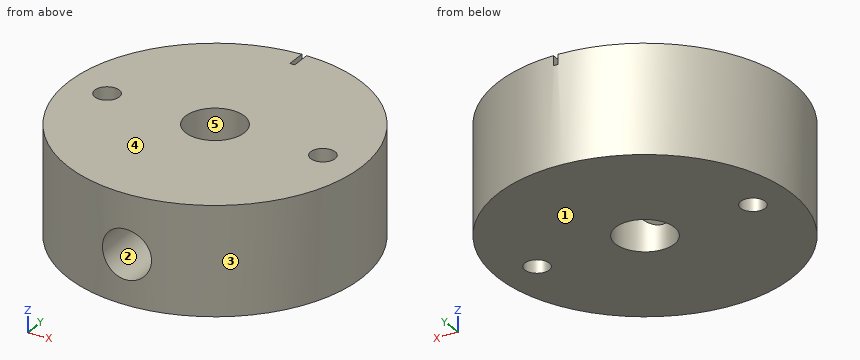
from build123d import *

# Parameters (mm, degrees)
CROQUIS1_R              = 15
CROQUIS1_R_2            = 3
SALIENTE_EXTRUIR1_DEPTH = 11
CORTAR_EXTRUIR1_START   = -1
CORTAR_EXTRUIR1_DEPTH   = 1
CROQUIS3_R              = 1.25
CORTAR_EXTRUIR2_DEPTH   = 24.895606291
CROQUIS4_R              = 2.5
CORTAR_EXTRUIR3_DEPTH   = 16


# Read off the part's stored shape, not the designer's step: Cortar-Extruir1
with BuildPart() as part:
    # Croquis1 → Saliente-Extruir1 (new body)
    with BuildSketch(Plane.XY):
        Circle(CROQUIS1_R)
        Circle(CROQUIS1_R_2, mode=Mode.SUBTRACT)
    extrude(amount=SALIENTE_EXTRUIR1_DEPTH)

    # Cortar-Extruir1 outline → Cortar-Extruir1 (cut)
    with BuildSketch(Plane.XY.offset(11).offset(CORTAR_EXTRUIR1_START)):
        with BuildLine():
            Line((-0.25, 14.997916522), (-0.25, 12.997916522))
            Line((-0.25, 12.997916522), (0.25, 12.997916522))
            Line((0.25, 12.997916522), (0.25, 14.997916522))
            ThreePointArc((0.25, 14.997916522), (0, 15), (-0.25, 14.997916522))
        make_face()
    extrude(amount=CORTAR_EXTRUIR1_DEPTH, mode=Mode.SUBTRACT)

    # Croquis3 → Cortar-Extruir2 (cut, through all)
    with BuildSketch(Plane.XY.offset(11)):
        with Locations((11, 0)):
            Circle(CROQUIS3_R)
        with Locations((-11, 0)):
            Circle(CROQUIS3_R)
    extrude(amount=-CORTAR_EXTRUIR2_DEPTH, mode=Mode.SUBTRACT)

    # Croquis4 → Cortar-Extruir3 (cut)
    with BuildSketch(Plane(origin=(0, 0, 0), x_dir=(1, 0, 0), z_dir=(0, 1, 0))):
        with Locations(Location((0, -5, 0), (0, 0, 270))):
            Circle(CROQUIS4_R)
    extrude(amount=-CORTAR_EXTRUIR3_DEPTH, mode=Mode.SUBTRACT)


solid = part.part
Build history of the part. All positions in model axes, mm. Face numbers are marked on the shaded views. A direction names the side the tool comes from. Coordinates: 2 decimals unless noted, no trailing zeros. Write each loop counter-clockwise with the first axis right and the second up, starting at its lowest first coordinate (ties: lowest second). Pieces come first, ordered by that corner, then holes.
(1) Cut at D-D on z = 5. List the corners of the cut face in (x, y).
(2) Mould opens along Y. For the marked faces 3, 4 and 5 say: pulls with the +Y half, pulls with the -Y half, needs draft (parallel to the pull), parting line crosses it, or undercut.
(3) Pin check, flat tips, straight feed: pin 1 Ø2 at (x, y) = (-9.5, 5) entering from -Z; pin 2 Ø0.8 at (y, z) = (14, 10.5) entering from -X; pin 3 Ø1.1 at (y, z) = (14, 10.5) entering from +X; pin 4 Ø5 at (y, z) = (4.5, 5) entering from +X. Stop position of each tip, or through.
(4) 3-axis set-ups, long thin cutter, end or side, ignore diameter. For the marked faces 1 and 2: which of +Z, -Z, +X, -X, +Y, -Y reach the whole face in a straight line?
(5) Cut at B-B on x = 1.5. List the corners of the cut face in (y, z).
(6) Cut at A-A on y = 0. List the corners of the cut face in (x, z).
(7) Cut at C-C on z = 9. List the corners of the cut face in (x, y).
(8) Drill centre lines: line 1 (Z direction, x = 0, y = -9.25); line 2 (X direction, y = -7.5, z = 5); line 3 (X direction, y = 1, z = 9.5). Where is each one in solid material? Low to high.
Working result:
1. outline: (-2.5, -14.79) - (-2.5, -1.66) arc R3 cw (long way) to (2.5, -1.66) - (2.5, -14.79) arc R15 ccw (long way) to start; hole circle Ø2.5 at (-11, 0); hole circle Ø2.5 at (11, 0)
2. face 3: parting line crosses it
2. face 4: needs draft
2. face 5: undercut
3. pin 1: stops at z = 0
3. pin 2: stops at x = -6.33
3. pin 3: stops at x = 6.64
3. pin 4: stops at x = 14.87
4. face 1: -Z, +X, -X, +Y, -Y
4. face 2: -Y
5. outline: (-14.92, 0) - (-2.6, 0) - (-2.6, 3) - (-14.92, 3) - close; (-14.92, 7) - (-2.6, 7) - (-2.6, 11) - (-14.92, 11) - close; (2.6, 0) - (14.92, 0) - (14.92, 11) - (2.6, 11) - close
6. outline: (-15, 0) - (-12.25, 0) - (-12.25, 11) - (-15, 11) - close; (-9.75, 0) - (-3, 0) - (-3, 11) - (-9.75, 11) - close; (3, 0) - (9.75, 0) - (9.75, 11) - (3, 11) - close; (12.25, 0) - (15, 0) - (15, 11) - (12.25, 11) - close
7. outline: circle Ø30 at (0, 0); hole circle Ø2.5 at (-11, 0); hole circle Ø6 at (0, 0); hole circle Ø2.5 at (11, 0)
8. line 1: z = 0 to 2.5, 7.5 to 11
8. line 2: x = -12.99 to -2.5, 2.5 to 12.99
8. line 3: x = -14.97 to -11.75, -10.25 to -2.83, 2.83 to 10.25, 11.75 to 14.97
